Here's how the part is built. I have some questions about the finished solid (model axes, mm). A direction names the side the tool comes from. Round coordinates to 2 decimals unless told otherwise and drop trailing zeros. Loops run counter-clockwise (first coordinate to the right, second up) from the corner with the lowest first, then second, coordinate; pieces in that order, holes last. Notation, with made-up numbers: M -40,83 L 4,83 A9 cw 4,96 Z; hole C -38,12 d6. An arc over 180 degrees is marked long. Use a Markdown table: item, result.
Autodesk Inventor part; units mm, degrees
ref_plane "YZ Plane" through (0, 0, 0) normal (1, 0, 0) x (0, 1, 0)
ref_plane "XZ Plane" through (0, 0, 0) normal (0, 1, 0) x (-1, 0, 0)
ref_plane "XY Plane" through (0, 0, 0) normal (0, 0, 1) x (1, 0, 0)
sketch "Sketch1" plane through (0, 0, 0) normal (0, 1, 0) x (-1, 0, 0)
  line L0 (0, 0) -> (50, 0)
  line L1 (50, 0) -> (50, -20)
  line L2 (50, -20) -> (0, -20)
  line L3 (0, -20) -> (0, 0)
  line L4 (50, -2) -> (53, -2)
  line L5 (53, -2) -> (53, -12)
  line L6 (53, -12) -> (50, -12)
  line L7 (25, -20) -> (25, 0) construction
  line L8 (0, -2) -> (-3, -2)
  line L9 (-3, -2) -> (-3, -12)
  line L10 (-3, -12) -> (0, -12)
  line L11 (50, -17) -> (42, -17)
  line L12 (42, -17) -> (42, -20)
  line L13 (8, -20) -> (8, -17)
  line L14 (8, -17) -> (0, -17)
  line L15 (30, -17) -> (20, -17)
  line L16 (20, -17) -> (20, -20)
  line L17 (20, -20) -> (30, -20)
  line L18 (30, -20) -> (30, -17)
  point P0 (25, -17)
  point P1 (30, -20)
  dimension "d0" = 20
  dimension "d1" = 50
  dimension "d2" = 2
  dimension "d3" = 10
  dimension "d4" = 3
  dimension "d7" = 8
  dimension "d8" = 3
  dimension "d9" = 10
extrude "Extrusion1" add sketch "Sketch1" along normal blind 3 contours L0 L1 L11 L12 L2 L18 L15 L16 L13 L14 L3 | L3 L10 L9 L8 | L4 L5 L6 L1
properties part number "soporte_base_parqueo"
Q1. Imagine slicing it at C-C, the plane x = -6. Please give me the cut outline in (y, z), then the cut area to 3 significant figures.
Return value:
| item | result |
|---|---|
| outline | M 0,-17 L 3,-17 L 3,0 L 0,0 Z |
| area | 51.0 mm^2 |
Q2. Imagine slicing it at B-B, the plane z = -13.75. Please give me the cut outline in (x, y).
Return value:
| item | result |
|---|---|
| outline | M -50,0 L 0,0 L 0,3 L -50,3 Z |
Q3. I need wall thicknesses on line 1 (X direction, y = 0.65, z = -18.75); line 2 (Z direction, x = -0.5, y = 2.3); line 3 (X direction, y = 1.25, z = -13.25). Which ranges of each line are inside material? Lowest first, please. Write a range as from..to.
Return value:
| item | result |
|---|---|
| line 1 | x = -42..-30, -20..-8 |
| line 2 | z = -17..0 |
| line 3 | x = -50..0 |
Q4. For faces 4 (the flat face through (-50, 1, -1)), 5 (the flat face through (-42, 1, -18)), 6 (the flat face through (-53, 1, -7)), 7 (the flat face through (-20, 1, -18)), 8 (the flat face through (-8, 1, -19)), which set-ups out of +Z, -Z, +X, -X, +Y, -Y let a thin tool reach every point of the face, with its end or its side?
Return value:
| item | result |
|---|---|
| face 4 | +Z, -X, +Y, -Y |
| face 5 | -Z, -X, +Y, -Y |
| face 6 | +Z, -Z, -X, +Y, -Y |
| face 7 | -Z, +Y, -Y |
| face 8 | -Z, +X, +Y, -Y |
Q5. Imagine slicing it at A-A, the plane y = 1.8. Please give me the cut outline in (x, z).
Return value:
| item | result |
|---|---|
| outline | M -53,-12 L -50,-12 L -50,-17 L -42,-17 L -42,-20 L -30,-20 L -30,-17 L -20,-17 L -20,-20 L -8,-20 L -8,-17 L 0,-17 L 0,-12 L 3,-12 L 3,-2 L 0,-2 L 0,0 L -50,0 L -50,-2 L -53,-2 Z |
Q6. We'd pull the mould along X, two halves only. Please class faces 1 (the flat face through (0, 1, -1)), 2 (the flat face through (-30, 1, -19)), 3 (the flat face through (1, 1, -2)): pulls with the +X half, pulls with the -X half, needs draft (parallel to the pull), parting line crosses it, or undercut.
Return value:
| item | result |
|---|---|
| face 1 | pulls with the +X half |
| face 2 | undercut |
| face 3 | needs draft |
Q7. Will these pins go through, and if not, where does the flat tip stop? P1, Ø3, axis at x = -45, z = -15.5, coming from the -Y side; P2, Ø0.9, axis at y = 2, z = -18.5, coming from the +X side; P3, Ø1.5, axis at x = 2, y = 2, coming from the -Z side; P4, Ø1.5, axis at y = 2, z = -18.5, coming from the -X side.
Return value:
| item | result |
|---|---|
| P1 | stops at y = 0 |
| P2 | stops at x = -8 |
| P3 | stops at z = -12 |
| P4 | stops at x = -42 |
